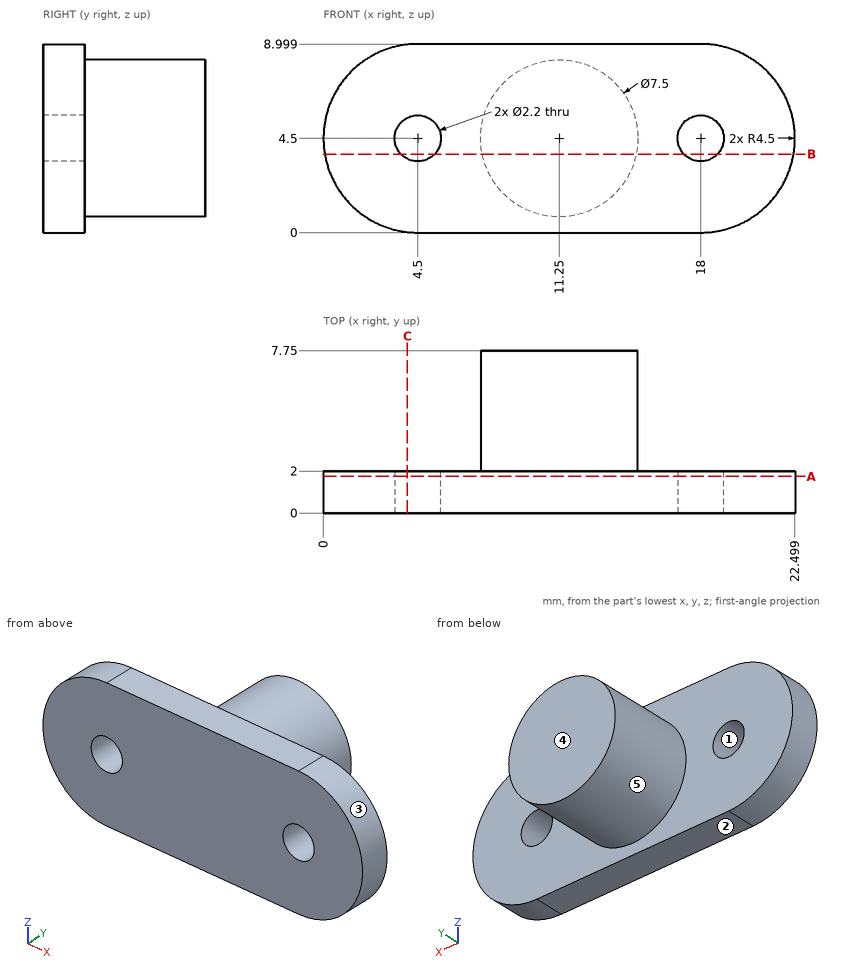
Design review of the part shown in the three views and the two pictorial views. Dimensions are in mm from the part's minimum x, y and z. A direction names the side the tool comes from. Coordinates: 2 decimals unless noted, no trailing zeros. Loops run counter-clockwise (first coordinate to the right, second up) from the corner with the lowest first, then second, coordinate; pieces in that order, holes last.
(1) Consider section A-A, the plane y = 1.75. Give the boundary of the cut face in (x, z).
Determined:
outline: (4.5, 0) - (18, 0) arc R4.5 ccw to (18, 9) - (4.5, 9) arc R4.5 ccw to start; hole circle Ø2.2 at (4.5, 4.5); hole circle Ø2.2 at (18, 4.5)
(2) Wall thickness on L1, parallel to X at y = 0.5, z = 5.25 (1 decimal); L2, parallel to Y at x = 3.75, z = 8; L3, parallel to Z at x = 11.25, y = 4: over which ranges is each line inside the solid? List them lowest first.
Determined:
L1: x = 0.1 to 3.7, 5.3 to 17.2, 18.8 to 22.4
L2: y = 0 to 2
L3: z = 0.75 to 8.25
(3) Draft analysis for pull direction X (two halves, no side actions). For the marked faces 1, 2 and 3, state which applies: +X half, -X half, draft (parallel to the pull), parting line (faces both ways), or undercut.
Determined:
face 1: undercut
face 2: draft
face 3: +X half
(4) Consider section B-B, the plane z = 3.75. Give the number of separate pieces and of enclosed holes in the cut face.
Determined:
separate pieces: 3
enclosed holes: 0
(5) Tool access review of the marked faces 4 and 5: name each direction out of +Z, -Z, +X, -X, +Y, -Y from which nothing blocks a thin tool from reaching the whole face with its end or side.
Determined:
face 4: +Z, -Z, +X, -X, +Y
face 5: +Y
(6) Consider section C-C, the plane x = 4. Give the boundary of the cut face in (y, z).
Determined:
outline: (0, 0.03) - (2, 0.03) - (2, 3.52) - (0, 3.52) - close; (0, 5.48) - (2, 5.48) - (2, 8.97) - (0, 8.97) - close
(7) Insertion check: P1, Ø1.5, axis at y = 5.5, z = 3.5, coming from the +X side. The pin has a flat end and moves straight along its axis. Give the tip position at first contact, or say it passes through.
Determined:
P1: stops at x = 14.99
